Check sheet for the modelled part. Datum: model origin and axes. Units: mm. A direction names the side the tool comes from. Coordinates: 2 decimals unless noted, no trailing zeros. Loops run counter-clockwise (first coordinate to the right, second up) from the corner with the lowest first, then second, coordinate; pieces in that order, holes last. Notation, with made-up numbers: (-9.75, -10) -> (8.25, -10) arc R18 ccw to (8.25, 6) -> close; hole circle Ø11 at (56.5, 58.5). An arc over 180 degrees is marked (long way). Use CSV: the item, a comma, the result in double quotes.
```python
from build123d import *

# Parameters (mm, degrees)
EXTRUDE_START            = 1.3
EXTRUDE_1_DEPTH          = 16
CUT_EXTRUDE_1_DEPTH      = 13.5
SKETCH_1_4_R             = 6.75
CUT_EXTRUDE_2_DEPTH      = 18.3
EXTRUDE_2_DEPTH          = 10
SKETCH_3_R               = 1.25
SKETCH_3_R_2             = 1.5
CUT_EXTRUDE_4_DEPTH      = 13.2
CUT_EXTRUDE_4_DEPTH_BACK = 4.8


with BuildPart() as part:
    # 草图1 → 凸台-拉伸1 (new body)
    with BuildSketch(Plane(origin=(0, 0, 0), x_dir=(0, 0, -1), z_dir=(1, 0, 0)).offset(EXTRUDE_START)):
        with BuildLine():
            Line((23.574545879, 54.705015226), (15.186652327, 42.269451638))
            ThreePointArc((15.186652327, 42.269451638), (18.559710691, 24.916570688), (35.912591641, 28.289629051))
            Line((35.912591641, 28.289629051), (44.300485193, 40.72519264))
            ThreePointArc((44.300485193, 40.72519264), (38.939692203, 55.131135816), (23.574545879, 54.705015226))
        make_face()
    extrude(amount=EXTRUDE_1_DEPTH)

    # 草图1<3> → 切除-拉伸1 (cut)
    with BuildSketch(Plane(origin=(0, 0, 0), x_dir=(0, 0, -1), z_dir=(1, 0, 0))):
        with BuildLine():
            ThreePointArc((20.461625434, 46.334508412), (37.873723753, 53.550772599), (37.705606944, 34.70329602))
            ThreePointArc((37.705606944, 34.70329602), (20.293508625, 27.487031833), (20.461625434, 46.334508412))
        make_face()
    extrude(amount=CUT_EXTRUDE_1_DEPTH, mode=Mode.SUBTRACT)

    # 草图1<4> → 切除-拉伸2 (cut, through all)
    with BuildSketch(Plane(origin=(0, 0, 0), x_dir=(0, 0, -1), z_dir=(1, 0, 0))):
        with Locations((31.554843944, 44.182648029)):
            Circle(SKETCH_1_4_R)
    extrude(amount=CUT_EXTRUDE_2_DEPTH, mode=Mode.SUBTRACT)

    # 草图2 → 凸台-拉伸2 (add)
    with BuildSketch(Plane.ZY.offset(-13.5)):
        with BuildLine():
            ThreePointArc((-20.461625434, 46.334508412), (-37.873723753, 53.550772599), (-37.705606944, 34.70329602))
            ThreePointArc((-37.705606944, 34.70329602), (-20.293508625, 27.487031833), (-20.461625434, 46.334508412))
        make_face()
        with BuildLine():
            ThreePointArc((-36.796785017, 35.31630415), (-20.852701529, 28.316069405), (-21.370447361, 45.721500282))
            ThreePointArc((-21.370447361, 45.721500282), (-37.314530849, 52.721735026), (-36.796785017, 35.31630415))
        make_face(mode=Mode.SUBTRACT)
    extrude(amount=EXTRUDE_2_DEPTH)

    # 草图3 → 切除-拉伸4 (cut, two sides)
    with BuildSketch(Plane.ZY.offset(-13.5)) as cut_extrude_4_sk:
        with Locations((-34.687312986, 33.626245342)):
            Circle(SKETCH_3_R)
        with Locations((-20.593674253, 43.132524701)):
            Circle(SKETCH_3_R)
        with Locations((-22.9057078, 27.783193072)):
            Circle(SKETCH_3_R_2)
        with Locations((-19.58955751, 30.019964685)):
            Circle(SKETCH_3_R_2)
    extrude(amount=CUT_EXTRUDE_4_DEPTH, mode=Mode.SUBTRACT)
    extrude(cut_extrude_4_sk.sketch, amount=-CUT_EXTRUDE_4_DEPTH_BACK, mode=Mode.SUBTRACT)


solid = part.part
```
1) Cross-section at A-A on z = -31.5. Record the boundary of the cut face in (x, y).
Answer below:
outline,"(1.3, 24.29) -> (17.3, 24.29) -> (17.3, 37.43) -> (13.5, 37.43) -> (13.5, 27.79) -> (3.5, 27.79) -> (3.5, 26.67) -> (1.3, 26.67) -> close; (1.3, 55.48) -> (3.5, 55.48) -> (3.5, 54.48) -> (13.5, 54.48) -> (13.5, 50.93) -> (17.3, 50.93) -> (17.3, 57.39) -> (1.3, 57.39) -> close"
2) Access from +Z, -Z, +X, -X, +Y, -Y to the whole of each face (thin tool, end or side, straight path). Record for faces 1 (the flat face through (1.3, 31, -37)), 2 (the cylindrical face through (2.385, 53.722, -37.613)).
Answer below:
face 1,"+Z, -Z, -X, +Y, -Y"
face 2,"-X"
3) Go/stop test with flat-tipped pins: pin 1 Ø2 at (y, z) = (43.13, -20.59) entering from +X; pin 2 Ø1 at (x, y) = (11.5, 39.5) entering from -Z; pin 3 Ø6 at (x, y) = (4.5, 40.5) entering from -Z; pin 4 Ø7.5 at (y, z) = (34.5, -27.5) entering from -X. Record where each tip stops, or that it passes through.
Answer below:
pin 1,"passes through"
pin 2,"stops at z = -43.81"
pin 3,"stops at z = -44.74"
pin 4,"stops at x = 13.5"
4) Thickness scan on line 1 along X through (y, z) = (35, -34); line 2 along Z through (x, y) = (10, 44); line 3 along Z through (x, y) = (4.25, 48). Record the ranges inside material, lowest first. Write a range as from..to.
Answer below:
line 1,"x = 13.5..17.3"
line 2,"z = -44.76..-41.85, -19.19..-16.35"
line 3,"z = -44.2..-41.12, -21.99..-19.05"
5) Cross-section at C-C on y = 48. Record the boundary of the cut face in (x, z), and give its area (3 significant figures).
Answer below:
outline,"(1.3, -44.2) -> (17.3, -44.2) -> (17.3, -37.12) -> (13.5, -37.12) -> (13.5, -41.12) -> (3.5, -41.12) -> (3.5, -42.19) -> (1.3, -42.19) -> close; (1.3, -20.92) -> (3.5, -20.92) -> (3.5, -21.99) -> (13.5, -21.99) -> (13.5, -25.99) -> (17.3, -25.99) -> (17.3, -19.05) -> (1.3, -19.05) -> close"
area,"122 mm²"
